Input: part model. Units: mm. Frame: model coordinates. A direction names the side the tool comes from. Coordinates: 2 decimals unless noted, no trailing zeros. Loops run counter-clockwise (first coordinate to the right, second up) from the corner with the lowest first, then second, coordinate; pieces in that order, holes last. Notation, with made-up numbers: (85, -38) -> (140, -38) arc R28 cw to (140, -1) -> close; hole circle Ø1 at (22.25, 85.25). An arc over 180 degrees is marked (long way). Put each result on its own line as item: value. Start each with the question number.
1) Cut plane B-B (z = 37). Return the cut outline in (x, y), plus the area to 3 significant figures.
2) Set-up query: faces 4 (the cylindrical face through (-0.49, 1.521, 59.443)), 5 (the flat face through (0, 0, 57)). Return all of +Z, -Z, +X, -X, +Y, -Y with unobstructed straight access to the full face (end or side cutting, diameter ignored); none if empty.
3) Pull-direction query (X, two-part tool) for faces 1 (the cylindrical face through (-32.544, 1.479, 64.492)), 2 (the flat face through (0, 2, 56.813)), 3 (the flat face through (0, 1, 64.813)); classes: pulls with the +X half, pulls with the -X half, needs draft (parallel to the pull), parting line crosses it, or undercut.
4) Contact query for flat-ended pins moving along their axis: P1, Ø1.5, axis at x = -64.5, y = 1.5, coming from the -Z side; P2, Ø1, axis at x = 16.5, y = 2, coming from the -Z side; P3, Ø0.7, axis at y = 2, z = -65, coming from the +X side. Output: stop coordinate, or through.
5) Cut plane C-C (y = 1.9). State how many separate pieces and enclosed holes the cut face has, plus the area to 3 significant figures.
6) Material intervals for L1, parallel to X at y = 1.55, z = 59; L2, parallel to Z at x = 18, y = 0.45; L3, parallel to X at y = 2.65, z = -16, sorted ascending.
7) Cut plane A-A (x = -18.5). Return the cut outline in (y, z).
from build123d import *

# Parameters (mm, degrees)
BOSS_EXTRUDE1_DEPTH = 3
SKETCH2_W           = 15
SKETCH2_H           = 3
SKETCH2_W_2         = 6
SKETCH2_H_2         = 15
SKETCH2_H_3         = 4
BOSS_EXTRUDE2_DEPTH = 3
CUT_EXTRUDE1_DEPTH  = 103.574363269
CUT_EXTRUDE2_DEPTH  = 103.574363269
FILLET1_R           = 1


with BuildPart() as part:
    # Sketch1 → Boss-Extrude1 (new body)
    with BuildSketch(Plane(origin=(0, 0, 0), x_dir=(1, 0, 0), z_dir=(0, 1, 0))):
        with BuildLine():
            Line((-30.029977361, -64.812867647), (30.029977361, -64.812867647))
            ThreePointArc((30.029977361, -64.812867647), (32.509837414, -64.500503794), (34.834773739, -63.582926471))
            ThreePointArc((34.834773739, -63.582926471), (0, 72.5), (-34.834773739, -63.582926471))
            ThreePointArc((-34.834773739, -63.582926471), (-32.509837414, -64.500503794), (-30.029977361, -64.812867647))
        make_face()
        with BuildLine():
            Line((-30.029977361, -59.812867647), (30.029977361, -59.812867647))
            ThreePointArc((30.029977361, -59.812867647), (31.269907388, -59.656685721), (32.43237555, -59.197897059))
            ThreePointArc((32.43237555, -59.197897059), (0, 67.5), (-32.43237555, -59.197897059))
            ThreePointArc((-32.43237555, -59.197897059), (-31.269907388, -59.656685721), (-30.029977361, -59.812867647))
        make_face(mode=Mode.SUBTRACT)
    extrude(amount=BOSS_EXTRUDE1_DEPTH)

    # Sketch2 → Boss-Extrude2 (add)
    with BuildSketch(Plane(origin=(0, 3, 0), x_dir=(1, 0, 0), z_dir=(0, 1, 0))):
        with Locations((0, -58.312867647)):
            Rectangle(SKETCH2_W, SKETCH2_H)
        with Locations((-64.5, 0)):
            Rectangle(SKETCH2_W_2, SKETCH2_H_2)
        with Locations((64.5, 0)):
            Rectangle(SKETCH2_W_2, SKETCH2_H_2)
        with Locations((0, 65.5)):
            Rectangle(SKETCH2_W, SKETCH2_H_3)
    extrude(amount=-BOSS_EXTRUDE2_DEPTH)

    # Sketch3 → Cut-Extrude1 (cut, through all)
    with BuildSketch(Plane(origin=(0, 3, 0), x_dir=(1, 0, 0), z_dir=(0, 1, 0))):
        with BuildLine():
            ThreePointArc((1.616415185, -63.268268373), (5.208836136, -60.842325617), (1.43798531, -58.704249242))
            ThreePointArc((1.43798531, -58.704249242), (-0.518832115, -59.450153065), (-2.604077426, -59.643178828))
            ThreePointArc((-2.604077426, -59.643178828), (-3.959545317, -60.885236313), (-2.717487833, -62.240704205))
            ThreePointArc((-2.717487833, -62.240704205), (-0.501795592, -62.548915084), (1.616415185, -63.268268373))
        make_face()
        with BuildLine():
            ThreePointArc((2.86579375, 65.637468158), (4.221261642, 66.879525642), (2.979204157, 68.234993534))
            ThreePointArc((2.979204157, 68.234993534), (0.457508066, 68.55960428), (-1.973827963, 69.303195854))
            ThreePointArc((-1.973827963, 69.303195854), (-5.470477452, 66.834714499), (-1.788525063, 64.652242401))
            ThreePointArc((-1.788525063, 64.652242401), (0.476176032, 65.439915463), (2.86579375, 65.637468158))
        make_face()
    extrude(amount=-CUT_EXTRUDE1_DEPTH, mode=Mode.SUBTRACT)

    # Sketch4 → Cut-Extrude2 (cut, through all)
    with BuildSketch(Plane(origin=(0, 3, 0), x_dir=(1, 0, 0), z_dir=(0, 1, 0))):
        with BuildLine():
            Line((-67.991984271, 1.667355653), (-66.410615041, 1.598311581))
            Line((-66.410615041, 1.598311581), (-67.139557844, 0.548042688))
            ThreePointArc((-67.139557844, 0.548042688), (-67.790591563, -0.111174979), (-68.626151234, -0.511490946))
            ThreePointArc((-68.626151234, -0.511490946), (-69.389235809, -5.060995376), (-65.394055237, -2.75473849))
            ThreePointArc((-65.394055237, -2.75473849), (-65.311299925, -1.831936022), (-64.921452747, -0.991440921))
            Line((-64.921452747, -0.991440921), (-64.156516626, 0.110687546))
            ThreePointArc((-64.156516626, 0.110687546), (-63.962986737, 2.747929937), (-66.179059274, 4.190678619))
            Line((-66.179059274, 4.190678619), (-67.878573864, 4.264881029))
            ThreePointArc((-67.878573864, 4.264881029), (-69.234041756, 3.022823544), (-67.991984271, 1.667355653))
        make_face()
        with BuildLine():
            Line((67.991984271, -1.667355653), (66.410615041, -1.598311581))
            Line((66.410615041, -1.598311581), (67.139557844, -0.548042688))
            ThreePointArc((67.139557844, -0.548042688), (67.790591563, 0.111174979), (68.626151234, 0.511490946))
            ThreePointArc((68.626151234, 0.511490946), (69.389235809, 5.060995376), (65.394055237, 2.75473849))
            ThreePointArc((65.394055237, 2.75473849), (65.311299925, 1.831936022), (64.921452747, 0.991440921))
            Line((64.921452747, 0.991440921), (64.156516626, -0.110687546))
            ThreePointArc((64.156516626, -0.110687546), (63.962986737, -2.747929937), (66.179059274, -4.190678619))
            Line((66.179059274, -4.190678619), (67.878573864, -4.264881029))
            ThreePointArc((67.878573864, -4.264881029), (69.234041756, -3.022823544), (67.991984271, -1.667355653))
        make_face()
    extrude(amount=-CUT_EXTRUDE2_DEPTH, mode=Mode.SUBTRACT)

    # Fillet1
    fillet1_edges = [part.edges().sort_by_distance(p)[0] for p in [
        (7.5, 1.5, 56.812867647),
        (7.5, 1.5, 59.812867647),
        (-7.5, 1.5, 59.812867647),
        (-7.5, 1.5, 56.812867647),
        (-67.082039325, 1.5, -7.5),
        (-67.082039325, 1.5, 7.5),
        (-61.5, 1.5, -7.5),
        (-61.5, 1.5, 7.5),
        (67.082039325, 1.5, 7.5),
        (67.082039325, 1.5, -7.5),
        (61.5, 1.5, 7.5),
        (61.5, 1.5, -7.5),
        (7.5, 1.5, -67.082039325),
        (7.5, 1.5, -63.5),
        (-7.5, 1.5, -67.082039325),
        (-7.5, 1.5, -63.5),
    ]]
    fillet(fillet1_edges, radius=FILLET1_R)


solid = part.part
Results found:
1. outline: (-62.35, 0) -> (-56.46, 0) -> (-56.46, 3) -> (-62.35, 3) -> close; (56.46, 0) -> (62.35, 0) -> (62.35, 3) -> (56.46, 3) -> close
1. area: 35.4 mm2
2. face 4: +Y, -Y
2. face 5: +Z, -Z, +X, -X, -Y
3. face 1: pulls with the -X half
3. face 2: undercut
3. face 3: needs draft
4. P1: stops at z = -34.53
4. P2: stops at z = -70.71
4. P3: stops at x = 32.81
5. separate pieces: 1
5. enclosed holes: 5
5. area: 2,320 mm2
6. L1: x = -42.13 to -32.79, -7.52 to 0.84, 4.31 to 7.52, 32.79 to 42.13
6. L2: z = -70.23 to -65.06, 59.81 to 64.81
6. L3: x = -70.71 to -65.58, 65.58 to 70.71
7. outline: (0, -70.1) -> (3, -70.1) -> (3, -64.92) -> (0, -64.92) -> close; (0, 59.81) -> (3, 59.81) -> (3, 64.81) -> (0, 64.81) -> close
